Geometry check sheet. Reference: the model listing, model coordinates, mm. Face numbers are marked on the shaded views. A direction names the side the tool comes from. Coordinates: 2 decimals unless noted, no trailing zeros. Loops run counter-clockwise (first coordinate to the right, second up) from the corner with the lowest first, then second, coordinate; pieces in that order, holes last. Notation, with made-up numbers: M -29.5,22 L -14.5,22 A20 cw -14.5,61 Z; hole C -34.5,-18.5 d4. An arc over 180 degrees is marked long. Use CSV: the item, a comma, the result in double quotes.
Autodesk Inventor part; units mm, degrees
ref_plane "YZ Plane" through (0, 0, 0) normal (1, 0, 0) x (0, 1, 0)
ref_plane "XZ Plane" through (0, 0, 0) normal (0, 1, 0) x (-1, 0, 0)
ref_plane "XY Plane" through (0, 0, 0) normal (0, 0, 1) x (1, 0, 0)
sketch "Skizze1" plane through (0, 0, 0) normal (0, 0, 1) x (1, 0, 0)
  line L0 (0, 0) -> (11, 0)
  line L1 (11, 0) -> (11, -6)
  line L2 (11, -6) -> (0, -6)
  line L3 (0, -6) -> (0, 0)
  line L4 (0, -6) -> (2, -6)
  line L5 (2, -6) -> (2, -11)
  line L6 (2, -11) -> (0, -11)
  line L7 (0, -11) -> (0, -6)
  line L8 (11, -6) -> (8.5, -6)
  line L9 (7.5, -6) -> (11, -10)
  line L10 (11, -10) -> (11, -6)
  dimension "d0" = 11
  dimension "d1" = 6
  dimension "d2" = 2
  dimension "d3" = 5
  dimension "d5" = 5.5
  dimension "d6" = 4
revolve "Umdrehung1" add sketch "Skizze1" angle 360 about axis through (0, 0, 0) along (1, 0, 0)
sketch "Skizze3" plane through (11, 0, 0) normal (1, 0, 0) x (0, 0, -1)
  circle A0 centre (0, 0) radius 10
  circle A1 centre (0, 0) radius 11
  circle A2 centre (0.009, 0) radius 2.675
  line L0 (-2.2058, 1.5) -> (2.2239, 1.5)
  line L1 (-2.2058, -1.5) -> (2.2239, -1.5)
  point P0 (17.2536, -1.634)
  dimension "d8" = 5.35
  dimension "d9" = 1.5
  dimension "d10" = 1.5
extrude "Extrusion1" cut sketch "Skizze3" against normal blind 8.5 contours A2 L1 L0
extrude "Extrusion2" cut sketch "Skizze3" against normal blind 1.7 contours L0 A2 | A2 L1
sketch "Skizze4" plane through (0, 0, 0) normal (-1, 0, 0) x (0, 0, 1)
  circle A0 centre (0, 0) radius 11
  circle A1 centre (0, 0) radius 6
  arc A2 (2.2058, -1.5) -> (2.2058, 1.5) centre (-0.009, 0) ccw
  arc A3 (-2.2239, -1.5) -> (2.2058, -1.5) centre (-0.009, 0) ccw
  arc A4 (-2.2239, 1.5) -> (-2.2239, -1.5) centre (-0.009, 0) ccw
  line L0 (2.2058, 1.5) -> (-2.2239, 1.5)
  line L1 (-2.2239, -1.5) -> (2.2058, -1.5)
  arc A5 (2.2058, 1.5) -> (-2.2239, 1.5) centre (-0.009, 0) ccw
  line L2 (-10.6271, -3.15) -> (10.6271, -3.15)
  line L3 (10.6271, -3.15) -> (10.6271, -2.84)
  line L4 (10.6271, -2.84) -> (-10.6271, -2.84)
  line L5 (-10.6271, -2.84) -> (-10.6271, -3.15)
  circle A6 centre (0, 0) radius 11
  dimension "d15" = 0.31
  dimension "d16" = 2.84
extrude "Extrusion3" cut sketch "Skizze4" against normal blind 6.5 contours L4 A1 L2 A0 | A0 L2 L5 | L3 L2 A0 | A0 L2 A1 L4 | L4 A1 L2
chamfer "Fase1" distance 1 angle 45 2 edges at (0, -2.84, 0) (0, -3.15, 0)
chamfer "Fase2" distance 0.3 angle 45 2 edges at (0, -11, 0) (0, 11, 0)
sketch "Skizze5" plane through (0, 0, 0) normal (0, 1, 0) x (-1, 0, 0)
  circle A0 centre (-4.5, 0) radius 1.8
  line L0 (0, 10.7) -> (0, -10.7)
  point P0 (0, 0)
  point P1 (0, -10.5406)
  point P2 (0, 10.5406)
  dimension "d25" = 3.6
  dimension "d26" = 4.5
extrude "Extrusion4" [suppressed]
properties part number "PullingWheel"
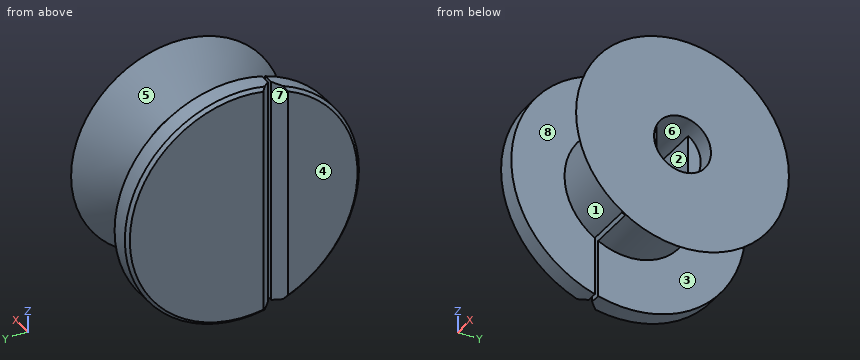
1. Section check A-A, the plane x = 5. Record the cut outline in (y, z) (3 decimals), plus the area to 3 significant figures.
The answers:
outline,"M -3.15,-5.107 L -3.15,5.107 A6 ccw Z; M -2.84,-5.285 A6 ccw long -2.84,5.285 Z; hole M -1.5,-2.224 A2.675 ccw 1.5,-2.224 L 1.5,2.206 A2.675 ccw -1.5,2.206 Z"
area,"94.7 mm^2"
2. Thickness scan on line 1 (Y direction, x = 6.25, z = -0.25); line 2 (Z direction, x = 7.25, y = 0); line 3 (X direction, y = -9, z = -5). Record the ranges inside material, lowest first. Write a range as [from, to].
The answers:
line 1,"[-5.99, -3.15], [-2.84, -1.5], [1.5, 5.99]"
line 2,"[-6, -2.68], [2.67, 6]"
line 3,"[0, 2]"
3. Set-up check for the marked faces 4, 5, 6, 7 and 8: record each of +Z, -Z, +X, -X, +Y, -Y from which the full face is reachable in a straight line by a thin tool's end or side.
The answers:
face 4,"+Z, -Z, -X, +Y, -Y"
face 5,"none"
face 6,"+X"
face 7,"+Z, -Z, -X"
face 8,"-Y"
4. Section check C-C, the plane x = 8.25. Record the cut outline in (y, z) (3 decimals).
The answers:
outline,"C 0,0 d13.714; hole M -1.5,-2.224 A2.675 ccw 1.5,-2.224 L 1.5,2.206 A2.675 ccw -1.5,2.206 Z"
5. Release check for a two-part mould opening along Y. For the marked faces 1, 2 and 3 record: +Y half, -Y half, draft (parallel to the pull), parting line (faces both ways), or undercut.
The answers:
face 1,"parting line"
face 2,"undercut"
face 3,"draft"
6. Gauge pin test, flat ends, axial feed: P1, Ø3.5, axis at x = 5.5, z = 0.5, coming from the -Y side; P2, Ø1, axis at x = 7.5, z = -3.5, coming from the +Y side; P3, Ø8, axis at y = -2.5, z = 4, coming from the -X side; P4, Ø0.6, axis at y = -2, z = 1, coming from the +X side. Record the tip position at first contact, or that the pin passes through.
The answers:
P1,"y = -6"
P2,"y = 5.63"
P3,"x = 0"
P4,"x = 9.3"
7. Section check B-B, the plane y = 0. Record the cut outline in (x, z), plus the area to 3 significant figures.
The answers:
outline,"M 0,-10.7 L 0.3,-11 L 2,-11 L 2,-6 L 7.5,-6 L 11,-10 L 11,-2.68 L 2.5,-2.68 L 2.5,2.67 L 11,2.67 L 11,10 L 7.5,6 L 2,6 L 2,11 L 0.3,11 L 0,10.7 Z"
area,"120 mm^2"
8. Section check D-D, the plane z = 0. Record the cut outline in (x, y).
The answers:
outline,"M 0,-10.7 L 0.3,-11 L 2,-11 L 2,-6 L 7.5,-6 L 11,-10 L 11,-2.67 L 9.3,-2.67 L 9.3,-1.5 L 2.5,-1.5 L 2.5,1.5 L 9.3,1.5 L 9.3,2.67 L 11,2.67 L 11,10 L 7.5,6 L 2,6 L 2,11 L 0.3,11 L 0,10.7 L 0,-1.84 L 1,-2.84 L 6.5,-2.84 L 6.5,-3.15 L 1,-3.15 L 0,-4.15 Z"
